```python
from build123d import *

# Parameters (mm, degrees)
SKETCH1_R                      = 10
SKETCH1_R_2                    = 2.5
BOSS_EXTRUDE1_DEPTH            = 5
BOSS_EXTRUDE4_DEPTH            = 10
SKETCH6_R                      = 0.75
CUT_EXTRUDE3_DEPTH             = 21
SKETCH7_R                      = 2
CUT_EXTRUDE4_DEPTH             = 2.5
SKETCH8_R                      = 2
CUT_EXTRUDE5_DEPTH             = 2.5
BOSS_EXTRUDE5_START            = -7.5
SKETCH10_R                     = 1.5
BOSS_EXTRUDE5_DEPTH            = 10.5
CUT_EXTRUDE6_REACH             = 12
SKETCH11_R                     = 0.5
CUT_EXTRUDE6_DIRECTION_2_REACH = 12
SKETCH12_R                     = 2.5
CUT_EXTRUDE7_DEPTH             = 2
CIRPATTERN1_COUNT              = 4
SKETCH13_R                     = 5.4
SKETCH13_R_2                   = 4.15
CUT_EXTRUDE8_DEPTH             = 2


with BuildPart() as part:
    # Sketch1 → Boss-Extrude1 (new body)
    with BuildSketch(Plane(origin=(0, 0, 0), x_dir=(1, 0, 0), z_dir=(0, 1, 0))):
        Circle(SKETCH1_R)
        Circle(SKETCH1_R_2, mode=Mode.SUBTRACT)
    extrude(amount=BOSS_EXTRUDE1_DEPTH)

    # Sketch5 → Boss-Extrude4 (add)
    with BuildSketch(Plane(origin=(0, 5, 0), x_dir=(1, 0, 0), z_dir=(0, 1, 0))):
        with BuildLine():
            Line((4.5, 8.93028555), (4.5, -8.93028555))
            ThreePointArc((4.5, -8.93028555), (10, 0), (4.5, 8.93028555))
        make_face()
        with BuildLine():
            Line((-4.5, 8.93028555), (-4.5, -8.93028555))
            ThreePointArc((-4.5, -8.93028555), (-10, 0), (-4.5, 8.93028555))
        make_face()
    extrude(amount=BOSS_EXTRUDE4_DEPTH)

    # Sketch6 → Cut-Extrude3 (cut, through all)
    with BuildSketch(Plane.ZY.offset(10)):
        with Locations((-5, 10)):
            Circle(SKETCH6_R)
        with Locations((5, 10)):
            Circle(SKETCH6_R)
    extrude(amount=-CUT_EXTRUDE3_DEPTH, mode=Mode.SUBTRACT)

    # Sketch7 → Cut-Extrude4 (cut)
    with BuildSketch(Plane.ZY.offset(10)):
        with Locations((-5, 10)):
            Circle(SKETCH7_R)
        with Locations((5, 10)):
            Circle(SKETCH7_R)
    extrude(amount=-CUT_EXTRUDE4_DEPTH, mode=Mode.SUBTRACT)

    # Sketch8 → Cut-Extrude5 (cut)
    with BuildSketch(Plane(origin=(10, 0, 0), x_dir=(0, 0, -1), z_dir=(1, 0, 0))):
        with Locations((-5, 10)):
            Circle(SKETCH8_R)
        with Locations((5, 10)):
            Circle(SKETCH8_R)
    extrude(amount=-CUT_EXTRUDE5_DEPTH, mode=Mode.SUBTRACT)

    # Sketch10 → Boss-Extrude5 (add)
    with BuildSketch(Plane.XY.offset(10).offset(BOSS_EXTRUDE5_START)):
        with Locations((0, 3.5)):
            Circle(SKETCH10_R)
    boss_extrude5 = extrude(amount=BOSS_EXTRUDE5_DEPTH)

    # Mirror1: Boss-Extrude5 across plane
    add(boss_extrude5.mirror(Plane.XY))

    # Sketch11 → Cut-Extrude6 (cut, up to next)
    with BuildSketch(Plane(origin=(0, 0, 0), x_dir=(0, 0, -1), z_dir=(1, 0, 0)), mode=Mode.PRIVATE) as cut_extrude6_sk1:
        with Locations((0, 10)):
            Circle(SKETCH11_R)
    cut_extrude6_tool1 = extrude(cut_extrude6_sk1.sketch, amount=-CUT_EXTRUDE6_REACH, mode=Mode.PRIVATE) & part.part
    add(cut_extrude6_tool1.solids().sort_by_distance((0, 10, 0))[0], mode=Mode.SUBTRACT)

    # Sketch11 → Cut-Extrude6 direction 2 (cut, up to next)
    with BuildSketch(Plane(origin=(0, 0, 0), x_dir=(0, 0, -1), z_dir=(1, 0, 0)), mode=Mode.PRIVATE) as cut_extrude6_direction_2_sk1:
        with Locations((0, 10)):
            Circle(SKETCH11_R)
    cut_extrude6_direction_2_tool1 = extrude(cut_extrude6_direction_2_sk1.sketch, amount=CUT_EXTRUDE6_DIRECTION_2_REACH, mode=Mode.PRIVATE) & part.part
    add(cut_extrude6_direction_2_tool1.solids().sort_by_distance((0, 10, 0))[0], mode=Mode.SUBTRACT)

    # Sketch12 → Cut-Extrude7 (cut)
    with BuildSketch(Plane.XZ):
        with Locations((-7.6, 0)):
            Circle(SKETCH12_R)
    cut_extrude7 = extrude(amount=-CUT_EXTRUDE7_DEPTH, mode=Mode.SUBTRACT)

    # CirPattern1: Cut-Extrude7 ×4 about axis
    cirpattern1_axis = Axis((0, 0, 0), (0, 1, 0))
    for i in range(1, CIRPATTERN1_COUNT):
        add(cut_extrude7.rotate(cirpattern1_axis, i * 360 / CIRPATTERN1_COUNT), mode=Mode.SUBTRACT)

    # Sketch13 → Cut-Extrude8 (cut)
    with BuildSketch(Plane.XZ):
        Circle(SKETCH13_R)
        Circle(SKETCH13_R_2, mode=Mode.SUBTRACT)
    extrude(amount=-CUT_EXTRUDE8_DEPTH, mode=Mode.SUBTRACT)


solid = part.part
```
Read the model definition and answer for the solid it produces. Units are mm, in the model's axes. A direction names the side the tool comes from. Give positions to 0.01 mm unless a question says otherwise; leave off trailing zeros. Loops run counter-clockwise (first coordinate to the right, second up) from the corner with the lowest first, then second, coordinate; pieces in that order, holes last.
Item 1: The mould has two halves that part along Y. Classify faces 6 (the cylindrical face through (-8, 10, 3)), 7 (the cylindrical face through (-1.5, 3.57, 11.42)), 8 (the cylindrical face through (-2.5, 1, -7.7)): released by +Y, released by -Y, zero draft, split by the parting line, or undercut.
Item 2: The part is cut by section D-D (y = 3.5). Write down the section's boundary in (x, z).
Item 3: Each of these flat-tipped pins is pushed along its axis until it touches: pin 1 Ø6 at (y, z) = (9, -9.5) entering from -X; pin 2 Ø1.8 at (y, z) = (10, 4) entering from +X; pin 3 Ø2.5 at (x, z) = (2, -4.5) entering from +Y; pin 4 Ø1.4 at (y, z) = (10, 5) entering from -X. Where does it stop, or does it pass through?
Item 4: The part is cut by section B-B (z = -5). Write down the section's boundary in (x, y), and give its area (3 significant figures).
Item 5: The part is cut by section C-C (x = 6.25). Write down the section's boundary in (y, z).
Item 6: For faces 1 (the cylindrical face through (-0.54, 2.46, 2.44)), 2 (the cylindrical face through (-6.02, 10.51, -5.55)), 3 (the cylindrical face through (3.85, 0.986, 3.786)), 4 (the cylindrical face through (8, 10, 3)), 5 (the flat face through (-7.5, 10, 4)), determine the directions among +Z, -Z, +X, -X, +Y, -Y from which every point of the face is accessible in a straight line to the end or side of a thin tool.
Item 7: Find the intervals of material crossed by line 1 along Y through (x, z) = (-6.75, 5); line 2 along Z through (x, y) = (-8.4, 10); line 3 along Y through (x, z) = (-7.35, 0), in increasing order.
Item 8: The part is cut by section A-A (y = 8.5). Write down the section's boundary in (x, z), and give its area (3 significant figures).
Taken from the geometry:
1. face 6: undercut
1. face 7: split by the parting line
1. face 8: zero draft
2. outline: (-1.5, -13) - (1.5, -13) - (1.5, -9.89) arc R10 ccw to (1.5, 9.89) - (1.5, 13) - (-1.5, 13) - (-1.5, 9.89) arc R10 ccw to (-1.5, -9.89) - close; hole circle Ø5 at (0, 0)
3. pin 1: stops at x = -7.59
3. pin 2: stops at x = 7.5
3. pin 3: stops at y = 5
3. pin 4: passes through
4. outline: (-8.66, 0) - (-2.04, 0) - (-2.04, 2) - (2.04, 2) - (2.04, 0) - (8.66, 0) - (8.66, 8) - (7.5, 8) - (7.5, 9.25) - (4.5, 9.25) - (4.5, 5) - (-4.5, 5) - (-4.5, 9.25) - (-7.5, 9.25) - (-7.5, 8) - (-8.66, 8) - close; (-8.66, 12) - (-7.5, 12) - (-7.5, 10.75) - (-4.5, 10.75) - (-4.5, 15) - (-8.66, 15) - close; (4.5, 10.75) - (7.5, 10.75) - (7.5, 12) - (8.66, 12) - (8.66, 15) - (4.5, 15) - close
4. area: 143 mm2
5. outline: (0, -7.81) - (15, -7.81) - (15, 7.81) - (0, 7.81) - (0, 2.1) - (2, 2.1) - (2, -2.1) - (0, -2.1) - close; hole circle Ø1.5 at (10, -5); hole circle Ø1.5 at (10, 5); hole circle Ø1 at (10, 0)
6. face 1: +Y, -Y
6. face 2: +X, -X
6. face 3: -Y
6. face 4: +X
6. face 5: -X
7. line 1: y = 0 to 9.25, 10.75 to 15
7. line 2: z = -3 to -0.5, 0.5 to 3
7. line 3: y = 2 to 9.5, 10.5 to 15
8. outline: (-9.3, -3.68) - (-7.5, -3.68) - (-7.5, -6.32) - (-7.75, -6.32) arc R10 ccw to (-4.5, -8.93) - (-4.5, 8.93) arc R10 ccw to (-7.75, 6.32) - (-7.5, 6.32) - (-7.5, 3.68) - (-9.3, 3.68) arc R10 ccw to start; (4.5, -8.93) arc R10 ccw to (7.75, -6.32) - (7.5, -6.32) - (7.5, -3.68) - (9.3, -3.68) arc R10 ccw to (9.3, 3.68) - (7.5, 3.68) - (7.5, 6.32) - (7.75, 6.32) arc R10 ccw to (4.5, 8.93) - close
8. area: 129 mm2
